from build123d import *

# Parameters (mm, degrees)
F0_W     = 76.2
F0_H     = 12.7
F0_H_2   = 6.35
F1_DEPTH = 45.72
F2_DEPTH = 20.32
F3_W     = 76.2
F3_H     = 19.05
F4_DEPTH = 10.16
F5_R     = 6.35
F5_R_2   = 12.7
F6_DEPTH = 76.201
F7_R     = 3.175


with BuildPart() as f1:
    # F0 (on Front) → F1 (new body)
    with BuildSketch(Plane.XZ):
        with Locations((38.1, 69.85)):
            Rectangle(F0_W, F0_H)
        with Locations((38.1, 60.325)):
            Rectangle(F0_W, F0_H_2)
        Polygon((0, 57.15), (0, 34.29), (76.2, 20.853884), (76.2, 57.15), align=None)
        Polygon((0, 34.29), (0, 25.4), (76.2, 11.963884), (76.2, 20.853884), align=None)
        Polygon((0, 25.4), (0, 0), (76.2, 0), (76.2, 11.963884), align=None)
    extrude(amount=-F1_DEPTH)

    # F0 (on Front) → F2 (join)
    with BuildSketch(Plane.XZ):
        with Locations((38.1, 69.85)):
            Rectangle(F0_W, F0_H)
        Polygon((0, 25.4), (0, 0), (76.2, 0), (76.2, 11.963884), align=None)
    extrude(amount=F2_DEPTH)

    # F3 (on face) → F4 (join)
    with BuildSketch(Plane.XZ.offset(20.32)):
        with Locations((38.1, 66.675)):
            Rectangle(F3_W, F3_H)
        Polygon((76.2, 20.853884), (0, 34.29), (0, 0), (76.2, 0), align=None)
    extrude(amount=F4_DEPTH)

    # F5 (on face) → F6 (cut, through all)
    with BuildSketch(Plane.XY.offset(76.2)):
        with Locations((19.05, -10.16)):
            Circle(F5_R)
        with Locations((57.15, -10.16)):
            Circle(F5_R)
        with Locations((38.1, 25.4)):
            Circle(F5_R_2)
    extrude(amount=-F6_DEPTH, mode=Mode.SUBTRACT)

    # F7
    f7_edges = [f1.edges().sort_by_distance(p)[0] for p in [
        (76.2, -30.48, 10.426942),
        (0, -30.48, 17.145),
        (76.2, 45.72, 38.1),
        (0, 45.72, 38.1),
        (76.2, -30.48, 66.675),
        (0, -30.48, 66.675),
    ]]
    fillet(f7_edges, radius=F7_R)


solid = f1.part
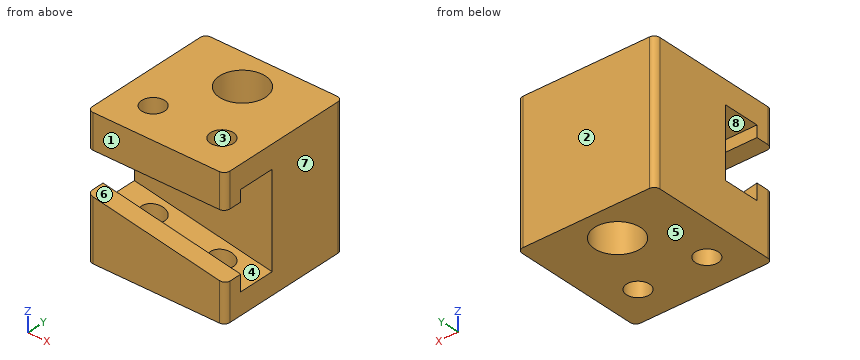
Read the model definition and answer for the solid it produces. Units are mm, in the model's axes. Face numbers are marked on the shaded views. A direction names the side the tool comes from. Round coordinates to 2 decimals unless told otherwise and drop trailing zeros. Write each loop counter-clockwise with the first axis right and the second up, starting at its lowest first coordinate (ties: lowest second). Pieces come first, ordered by that corner, then holes.
1. The part is cut by section B-B, the plane x = 46. Determine the outline of the cut face in (y, z).
2. Which of the six approach directions +Z, -Z, +X, -X, +Y, -Y give full straight-line access (tool end or side, diameter ignored) to the marked faces 4, 5, 6, 7 and 8?
3. Straight lines are drawn through the part: L1, parallel to X at y = -10.16, z = 6.25; L2, parallel to Y at x = 24, z = 29.5; L3, parallel to Y at x = 57, z = 10. For each, find the intervals that lie inside material, in ascending order.
4. The part is cut by section A-A, the plane z = 9. Determine the outline of the cut face in (x, y) (3 decimals).
5. Determine the mould class of the marked faces 1, 2 and 3 for opening direction Y: pulls with the +Y half, pulls with the -Y half, needs draft (parallel to the pull), parting line crosses it, or undercut.
6. The part is cut by section C-C, the plane y = 25.4. Determine the outline of the cut face in (x, z).
7. The part is cut by section D-D, the plane y = -10.16. Determine the outline of the cut face in (x, z), then the cut area to 3 significant figures.
Values:
1. outline: (-30.48, 0) - (15.46, 0) - (15.46, 76.2) - (-30.48, 76.2) - (-30.48, 57.15) - (-20.32, 57.15) - (-20.32, 63.5) - (0, 63.5) - (0, 17.29) - (-20.32, 17.29) - (-20.32, 26.18) - (-30.48, 26.18) - close; (35.34, 0) - (45.72, 0) - (45.72, 76.2) - (35.34, 76.2) - close
2. face 4: +X
2. face 5: -Z, +X, -X, +Y, -Y
2. face 6: +X, -Y
2. face 7: +Z, -Z, +X, +Y, -Y
2. face 8: +X, -X
3. L1: x = 0 to 12.7, 25.4 to 50.8, 63.5 to 76.2
3. L2: y = -30.48 to -20.32, 0 to 45.72
3. L3: y = -30.48 to -16.51, -3.81 to 45.72
4. outline: (0, -27.305) arc R3.175 ccw to (3.175, -30.48) - (73.025, -30.48) arc R3.175 ccw to (76.2, -27.305) - (76.2, 42.545) arc R3.175 ccw to (73.025, 45.72) - (3.175, 45.72) arc R3.175 ccw to (0, 42.545) - close; hole circle Ø12.7 at (19.05, -10.16); hole circle Ø25.4 at (38.1, 25.4); hole circle Ø12.7 at (57.15, -10.16)
5. face 1: pulls with the -Y half
5. face 2: pulls with the +Y half
5. face 3: undercut
6. outline: (0, 0) - (25.4, 0) - (25.4, 76.2) - (0, 76.2) - close; (50.8, 0) - (76.2, 0) - (76.2, 76.2) - (50.8, 76.2) - close
7. outline: (0, 0) - (12.7, 0) - (12.7, 23.16) - (0, 25.4) - close; (0, 63.5) - (12.7, 63.5) - (12.7, 76.2) - (0, 76.2) - close; (25.4, 0) - (50.8, 0) - (50.8, 16.44) - (25.4, 20.92) - close; (25.4, 63.5) - (50.8, 63.5) - (50.8, 76.2) - (25.4, 76.2) - close; (63.5, 0) - (76.2, 0) - (76.2, 11.96) - (63.5, 14.2) - close; (63.5, 63.5) - (76.2, 63.5) - (76.2, 76.2) - (63.5, 76.2) - close
7. area: 1,590 mm2
